Work out the finished part from the listing and answer in its coordinate system (mm). A direction names the side the tool comes from. Coordinates: 2 decimals unless noted, no trailing zeros. Loops run counter-clockwise (first coordinate to the right, second up) from the corner with the lowest first, then second, coordinate; pieces in that order, holes last. Notation, with made-up numbers: (82.5, 84) -> (105.5, 84) arc R24 cw to (105.5, 103) -> close; hole circle Ø1 at (53, 64.25). An arc over 180 degrees is marked (long way). Use a Markdown table: item, result.
Solid Edge part; units mm, degrees
sketch "Sketch1" plane through (0, 0, 0) normal (0, 0, 1) x (1, 0, 0)
  line L0 (0, 30) -> (120, 30)
  line L1 (120, 30) -> (120, -170)
  line L2 (120, -170) -> (75, -170)
  line L3 (75, -170) -> (75, 0)
  line L4 (75, 0) -> (0, 0)
  line L5 (0, 0) -> (0, 30)
  dimension "D1" = 120
  dimension "D2" = 120
extrude "Protrusion1" add sketch "Sketch1" against normal blind 20
hole "Hole1" at (120, -150, -10) direction (-1, 0, 0) diameter 6 end up to next
hole "Hole2" at (120, -130, -10) direction (-1, 0, 0) diameter 6 end up to next
fillet "Avrundning" radius 7 17 edges at (60, 30, 0) (120, -70, 0) (75, -85, 0) (37.5, 0, 0) (97.5, -170, 0) (75, -170, -10) (120, -170, -10) (97.5, -170, -20) (75, -85, -20) (120, -70, -20) (37.5, 0, -20) (0, 15, -20) (0, 0, -10) (0, 30, -10) (0, 15, 0) (60, 30, -20) (120, 30, -10)
properties material "Aluminum, 1060"
Q1. Section C-C on x = 62.5 is taken. Determine the outline of the cut face in (y, z), and give its area (3 significant figures).
Solved:
| item | result |
|---|---|
| outline | (0, -13) arc R7 ccw to (7, -20) -> (23, -20) arc R7 ccw to (30, -13) -> (30, -7) arc R7 ccw to (23, 0) -> (7, 0) arc R7 ccw to (0, -7) -> close |
| area | 558 mm² |
Q2. Determine the mould class of faces 1 (the cylindrical face through (117.9, -71.3, -18)), 2 (the cylindrical face through (2, 27.9, -10)), 3 (the cylindrical face through (98, -127, -10)) for opening direction Y: pulls with the +Y half, pulls with the -Y half, needs draft (parallel to the pull), parting line crosses it, or undercut.
Solved:
| item | result |
|---|---|
| face 1 | needs draft |
| face 2 | pulls with the +Y half |
| face 3 | undercut |
Q3. Section D-D on y = -109.5 is taken. Determine the outline of the cut face in (x, z), and give its area (3 significant figures).
Solved:
| item | result |
|---|---|
| outline | (75, -13) arc R7 ccw to (82, -20) -> (113, -20) arc R7 ccw to (120, -13) -> (120, -7) arc R7 ccw to (113, 0) -> (82, 0) arc R7 ccw to (75, -7) -> close |
| area | 858 mm² |
Q4. For faces 4 (the flat face through (84, -48, 0)), 5 (the flat face through (0, 15, -10)), 6 (the flat face through (41, 0, -10)), 7 (the cylindrical face through (77, -76.8, -2.1)), 8 (the cylindrical face through (77.1, -76.8, -18)), determine the directions among +Z, -Z, +X, -X, +Y, -Y from which every point of the face is accessible in a straight line to the end or side of a thin tool.
Solved:
| item | result |
|---|---|
| face 4 | +Z, +X, -X, +Y, -Y |
| face 5 | +Z, -Z, -X, +Y, -Y |
| face 6 | +Z, -Z, -X, -Y |
| face 7 | +Z, -X, -Y |
| face 8 | -Z, -X, -Y |
Q5. Given pin 1 Ø1.8 at (x, z) = (40, -10.5) entering from -Y; pin 2 Ø6 at (y, z) = (-119, -5) entering from -X; pin 3 Ø5.5 at (y, z) = (-130, -10) entering from +X; pin 4 Ø5 at (x, z) = (73.5, -8) entering from -Y, each flat-ended and moving along its own axis, determine where each tip first touches the part or whether it passes through.
Solved:
| item | result |
|---|---|
| pin 1 | y = 0 |
| pin 2 | x = 75 |
| pin 3 | through |
| pin 4 | y = -166.61 |
Q6. Consider line 1 (Y direction, x = 88, z = -10); line 2 (Z direction, x = 102, y = -150); line 3 (Y direction, x = 52.5, z = -10.5). Determine where each line is inside the solid, lowest interval first. Write a range as [from, to].
Solved:
| item | result |
|---|---|
| line 1 | [-170, -153], [-147, -133], [-127, 30] |
| line 2 | [-20, -13], [-7, 0] |
| line 3 | [0, 30] |
Q7. Section A-A on z = -10 is taken. Determine the outline of the cut face in (x, y), and give its area (3 significant figures).
Solved:
| item | result |
|---|---|
| outline | (0, 7) arc R7 ccw to (7, 0) -> (75, 0) -> (75, -127) -> (120, -127) -> (120, 23) arc R7 ccw to (113, 30) -> (7, 30) arc R7 ccw to (0, 23) -> close; (75, -163) arc R7 ccw to (82, -170) -> (113, -170) arc R7 ccw to (120, -163) -> (120, -153) -> (75, -153) -> close; (75, -147) -> (120, -147) -> (120, -133) -> (75, -133) -> close |
| area | 10,700 mm² |
